from build123d import *

# Parameters (mm, degrees)
SKETCH1_W                = 9
SKETCH1_H                = 11
SKETCH1_R                = 3.1
BOSS_EXTRUDE1_DEPTH      = 14
CUT_EXTRUDE1_DEPTH       = 10.8
BOSS_EXTRUDE2_DEPTH      = 1
SKETCH4_R                = 1
BOSS_EXTRUDE3_DEPTH      = 11.6
FILLET1_R                = 1
SKETCH5_R                = 0.5
BOSS_EXTRUDE4_DEPTH      = 0.01
BOSS_EXTRUDE4_DEPTH_BACK = 0.33
SKETCH6_R                = 0.5
BOSS_EXTRUDE5_DEPTH      = 0.01
BOSS_EXTRUDE5_DEPTH_BACK = 0.33
SKETCH8_R                = 0.5
BOSS_EXTRUDE6_DEPTH      = 0.33
FILLET2_R                = 0.1


with BuildPart() as part:
    # Sketch1 → Boss-Extrude1 (new body)
    with BuildSketch(Plane.XY):
        Rectangle(SKETCH1_W, SKETCH1_H)
        with Locations((0, 0.65)):
            Circle(SKETCH1_R, mode=Mode.SUBTRACT)
    extrude(amount=-BOSS_EXTRUDE1_DEPTH)

    # Sketch2 → Cut-Extrude1 (cut)
    with BuildSketch(Plane(origin=(0, 0, -14), x_dir=(-1, 0, 0), z_dir=(0, 0, -1))):
        with BuildLine():
            Line((-4.5, 5.5), (4.5, 5.5))
            Line((4.5, 5.5), (4.5, 1.15))
            Line((4.5, 1.15), (4.2, 1.15))
            ThreePointArc((4.2, 1.15), (0, 5), (-4.2, 1.15))
            Line((-4.2, 1.15), (-4.5, 1.15))
            Line((-4.5, 1.15), (-4.5, 5.5))
        make_face()
    extrude(amount=-CUT_EXTRUDE1_DEPTH, mode=Mode.SUBTRACT)

    # Sketch3 → Boss-Extrude2 (add)
    with BuildSketch(Plane(origin=(0, 0, -14), x_dir=(-1, 0, 0), z_dir=(0, 0, -1))):
        with BuildLine():
            Line((-4.5, 1.15), (-4.5, -5.5))
            Line((-4.5, -5.5), (4.5, -5.5))
            Line((4.5, -5.5), (4.5, 1.15))
            Line((4.5, 1.15), (4.2, 1.15))
            ThreePointArc((4.2, 1.15), (0, 5), (-4.2, 1.15))
            Line((-4.2, 1.15), (-4.5, 1.15))
        make_face()
    extrude(amount=-BOSS_EXTRUDE2_DEPTH)

    # Sketch4 → Boss-Extrude3 (add)
    with BuildSketch(Plane.XY.offset(-13)):
        with Locations((0, 0.65)):
            Circle(SKETCH4_R)
    extrude(amount=BOSS_EXTRUDE3_DEPTH)

    # Fillet1
    fillet1_edges = [part.edges().sort_by_distance(p)[0] for p in [
        (-1, 0.65, -1.4),
    ]]
    fillet(fillet1_edges, radius=FILLET1_R)

    # Sketch5 → Boss-Extrude4 (add, two sides)
    with BuildSketch(Plane(origin=(0, 0, -14), x_dir=(-1, 0, 0), z_dir=(0, 0, -1))) as boss_extrude4_sk:
        with BuildLine():
            Line((1.5, 2.472875656), (-1.5, 2.472875656))
            ThreePointArc((-1.5, 2.472875656), (-2, 1.15), (-1.5, -0.172875656))
            Line((-1.5, -0.172875656), (-1.5, -4.35))
            ThreePointArc((-1.5, -4.35), (-1.456066017, -4.456066017), (-1.35, -4.5))
            Line((-1.35, -4.5), (-1.315, -4.5))
            ThreePointArc((-1.315, -4.5), (-1.208933983, -4.543933983), (-1.165, -4.65))
            Line((-1.165, -4.65), (-1.165, -7.835))
            ThreePointArc((-1.165, -7.835), (0, -9), (1.165, -7.835))
            Line((1.165, -7.835), (1.165, -4.65))
            ThreePointArc((1.165, -4.65), (1.208933983, -4.543933983), (1.315, -4.5))
            Line((1.315, -4.5), (1.35, -4.5))
            ThreePointArc((1.35, -4.5), (1.456066017, -4.456066017), (1.5, -4.35))
            Line((1.5, -4.35), (1.5, -0.172875656))
            ThreePointArc((1.5, -0.172875656), (2, 1.15), (1.5, 2.472875656))
        make_face()
        with Locations((0, -7.835)):
            Circle(SKETCH5_R, mode=Mode.SUBTRACT)
    extrude(amount=BOSS_EXTRUDE4_DEPTH)
    extrude(boss_extrude4_sk.sketch, amount=-BOSS_EXTRUDE4_DEPTH_BACK)

    # Sketch6 → Boss-Extrude5 (add, two sides)
    with BuildSketch(Plane(origin=(4.5, 0, 0), x_dir=(0, 0, -1), z_dir=(1, 0, 0))) as boss_extrude5_sk:
        with BuildLine():
            Line((11.85, -7.925), (11.85, -1.5))
            Line((11.85, -1.5), (9.18, -1.5))
            Line((9.18, -1.5), (9.18, -4.1))
            Line((9.18, -4.1), (9.7, -4.1))
            Line((9.7, -4.1), (9.7, -7.925))
            ThreePointArc((9.7, -7.925), (10.775, -9), (11.85, -7.925))
        make_face()
        with Locations((10.775, -7.925)):
            Circle(SKETCH6_R, mode=Mode.SUBTRACT)
    extrude(amount=BOSS_EXTRUDE5_DEPTH)
    extrude(boss_extrude5_sk.sketch, amount=-BOSS_EXTRUDE5_DEPTH_BACK)

    # Sketch8 → Boss-Extrude6 (add)
    with BuildSketch(Plane(origin=(0, 0, -7.2), x_dir=(-1, 0, 0), z_dir=(0, 0, -1))):
        with BuildLine():
            Line((-1.165, -5.5), (1.165, -5.5))
            Line((1.165, -5.5), (1.165, -7.835))
            ThreePointArc((1.165, -7.835), (0, -9), (-1.165, -7.835))
            Line((-1.165, -7.835), (-1.165, -5.5))
        make_face()
        with Locations((0, -7.835)):
            Circle(SKETCH8_R, mode=Mode.SUBTRACT)
    extrude(amount=BOSS_EXTRUDE6_DEPTH)

    # Fillet2
    fillet2_edges = [part.edges().sort_by_distance(p)[0] for p in [
        (4.35, 1.15, -14),
        (-4.35, 1.15, -14),
        (-3.1, 0.65, 0),
        (4.5, 3.325, -3.2),
        (-4.5, 3.325, -3.2),
        (-4.5, -2.175, -14),
        (-2.8325, -5.5, -14),
        (2.8325, -5.5, -14),
        (4.5, -2.175, -14),
        (4.5, 1.15, -8.6),
        (4.2, 1.15, -8.6),
        (-4.2, 1.15, -8.6),
        (-4.5, 1.15, -8.6),
        (0, 5, -3.2),
        (0, 5, -14),
        (0, 5.5, -3.2),
        (0, 5.5, 0),
        (4.5, 0, 0),
        (-4.5, 0, 0),
        (-4.5, -5.5, -7),
        (0, -5.5, 0),
        (4.5, -5.5, -4.85),
        (-4.5, 5.5, -1.6),
        (4.5, 5.5, -1.6),
    ]]
    fillet(fillet2_edges, radius=FILLET2_R)


solid = part.part
Check sheet for the modelled part. Datum: model origin and axes. Units: mm. A direction names the side the tool comes from. Round coordinates to 2 decimals unless told otherwise and drop trailing zeros. Loops run counter-clockwise (first coordinate to the right, second up) from the corner with the lowest first, then second, coordinate; pieces in that order, holes last. Notation, with made-up numbers: M -22.5,-18 L 17.5,-18 A9 ccw 17.5,-2 Z; hole C 16,34 d10. An arc over 180 degrees is marked long. One line per item, written item: value.
(1) Access from +Z, -Z, +X, -X, +Y, -Y to the whole of each face (thin tool, end or side, straight path). Record for faces 1 (the face through (4.17, -7, -11)), 2 (the face through (1, 5.2, -3.2)), 3 (the face through (1.43, -2.1, -6.46)).
Computed values:
face 1: +Z, -Z, -X, -Y
face 2: -Z, +Y
face 3: +Z
(2) Depth check by flat-ended pin: pin 1 Ø2 at (x, y) = (-2, 4) entering from -Z; pin 2 Ø3 at (y, z) = (-3.5, -5.5) entering from +X; pin 3 Ø1.5 at (x, z) = (-1, -11.5) entering from +Y. Enter the tip coordinate at first touch or a pass-through.
Computed values:
pin 1: stops at z = -14
pin 2: stops at x = 4.5
pin 3: stops at y = 4.99
(3) Sectioned sample at A-A, the plane z = -9.5. Count the separate pieces of the cut face and the enclosed holes in it, then the cut area to 3 significant figures.
Computed values:
separate pieces: 2
enclosed holes: 1
area: 57.7 mm^2
(4) Sectioned sample at B-B, the plane z = -3.5. Record the cut outline in (x, y).
Computed values:
outline: M -4.5,-5.4 A0.1 ccw -4.4,-5.5 L 4.4,-5.5 A0.1 ccw 4.5,-5.4 L 4.5,1.05 A0.1 ccw 4.4,1.15 L 4.29,1.15 A0.1 cw 4.19,1.24 A4.22 ccw -4.19,1.24 A0.1 cw -4.29,1.15 L -4.4,1.15 A0.1 ccw -4.5,1.05 Z; C 0,0.65 d2; hole C 0,0.65 d6.2
(5) Thickness scan on line 1 (Y direction, x = 0.5, z = -2); line 2 (Y direction, x = 0.25, z = -8); line 3 (Z direction, x = -2.25, y = 3). Record the ranges inside material, lowest first.
Computed values:
line 1: y = -5.5 to -2.41, -0.12 to 1.42, 3.71 to 5.5
line 2: y = -5.5 to -2.44, -0.32 to 1.62, 3.74 to 4.99
line 3: z = -14 to 0
(6) Release check for a two-part mould opening along Z. For faces 4 (the face through (4.34, -7.43, -10.71)), 5 (the face through (4.5, -1, -5)), 6 (the face through (0, -5.5, -7)), 7 (the face through (2, 0, -14)) record: +Z half, -Z half, draft (parallel to the pull), parting line (faces both ways), or undercut.
Computed values:
face 4: undercut
face 5: draft
face 6: undercut
face 7: -Z half
